Could you check a few things on this model? Use its own coordinates, in mm. A direction names the side the tool comes from. Give positions to 0.01 mm unless a question says otherwise; leave off trailing zeros. Loops run counter-clockwise (first coordinate to the right, second up) from the corner with the lowest first, then second, coordinate; pieces in that order, holes last. Notation, with made-up numbers: M 19,84.5 L 47,84.5 A18 ccw 47,117.5 Z; hole C 24,0 d2. An arc over 180 degrees is marked long. Answer in a Markdown table with one row per item. Add a question column.
Autodesk Inventor part; units mm, degrees
ref_plane "Work Plane1" through (29, 0, 0) normal (0, -1, 0) x (1, 0, 0)
ref_plane "YZ Plane" through (0, 0, 0) normal (1, 0, 0) x (0, 1, 0)
ref_plane "XZ Plane" through (0, 0, 0) normal (0, 1, 0) x (-1, 0, 0)
sketch "Sketch1" plane through (0, 0, 0) normal (0, 0, 1) x (1, 0, 0)
  line L0 (0.2879, 0) -> (6.35, 0)
  line L1 (6.35, 0) -> (6.35, 2.413)
  line L2 (6.35, 2.413) -> (2.1084, 2.413)
  line L3 (2.1084, 2.413) -> (0.0001, 2.413)
  line L4 (0.0001, 2.413) -> (0, 2.413)
  line L5 (0, 2.413) -> (0, 4.5847)
  line L6 (0, 4.5847) -> (-2.5654, 4.5847)
  line L7 (-2.5654, 4.5847) -> (-2.5654, 1.8624)
  line L8 (-2.5654, 1.8624) -> (-0.7874, 1.8624)
  line L9 (-0.7874, 1.8624) -> (0.2879, 0)
  line L10 (-4.3485, 0) -> (8.1331, 0)
  line L11 (0, -0.9169) -> (0, 5.5016)
  line L12 (2.1084, 2.413) -> (0, 2.413) construction
  dimension "d1" = 4.2416
  dimension "d2" = 2.1083
  dimension "d3" = 2.5654
  dimension "d4" = 1.778
  dimension "d5" = 60
  dimension "d6" = 4.826
  dimension "d7" = 4.826
  dimension "d8" = 3.7248
  dimension "d9" = 9.1694
  dimension "d26" = 6.35
revolve "Body" add sketch "Sketch1" angle 360 about axis through (0.2879, 0, 0) along (1, 0, 0) contours L9 L11 L3 L2 L1 L0 | L9 L8 L7 L6 L5 L11
sketch "Sketch2" plane through (-2.5654, 0, 0) normal (-1, 0, 0) x (0, 0, 1)
  circle A0 centre (0, 0) radius 1.8624
  line L0 (0, -6.4186) -> (0, 6.4186)
  line L1 (-6.4186, 0) -> (6.4186, 0)
  line L2 (1.8624, 0) -> (0.9312, -1.6129)
  line L3 (0.9312, -1.6129) -> (-0.9312, -1.6129)
  line L4 (-0.9312, -1.6129) -> (-1.8624, 0)
  line L5 (-1.8624, 0) -> (-0.9312, 1.6129)
  line L6 (-0.9312, 1.6129) -> (0.9312, 1.6129)
  line L7 (0.9312, 1.6129) -> (1.8624, 0)
  point P0 (0, 0)
extrude "Slot" add sketch "Sketch2" against normal up to next contours L7 A0 | A0 L2 | L6 L0 A0 | A0 L0 L3 | L0 L6 A0 | A0 L3 L0 | L4 A0 | A0 L5
fillet "Fillet1" radius 2.0574 1 edges at (-2.5654, -4.5847, 0)
thread "Thread"
chamfer "Chamfer1" distance 0.4724 distance2 0.4724 1 edges at (6.35, -2.413, 0) measured on face at (6.35, -0.2686, 0.7084)
ref_plane "Work Plane1" through (29, 0, 0) normal (0, -1, 0) x (1, 0, 0)
fillet "Fillet2" radius 0.1 1 edges at (0.0001, -2.413, 0)
equation "\"d30\" = R"
equation "\"d17\" = RR"
equation "\"d13\" = GEL"
equation "\"d15\" = -0.5 * SPD + 0.5 * GD"
equation "\"d16\" = GUL"
equation "\"d1\" = GEL"
equation "\"d3\" = KOH"
equation "\"d4\" = INTI"
equation "\"d6\" = GD"
equation "\"d7\" = BDM"
equation "\"d8\" = 1.1547 * SW"
equation "\"d9\" = KOD"
equation "\"d26\" = NLG"
equation "\"GD\" = NND"
equation "\"NLG\" = 6.35"
equation "\"GEL\" = 4.2416"
equation "\"KOD\" = 9.1694"
equation "\"KOH\" = 2.5654"
equation "\"INTI\" = 1.778"
equation "\"GAL\" = 2.1082"
equation "\"GUL\" = 0.47244"
equation "\"BDM\" = NND"
equation "\"SW\" = 3.2258"
equation "\"RR\" = 2.0574"
equation "\"SPD\" = 3.88112"
equation "\"R\" = 0.1"
equation "\"TOA\" = 30deg"
equation "\"GD1\" = SPD"
equation "\"THREADDIA\" = 4.826"
equation "\"KOH1\" = 0.508"
equation "\"NND\" = 4.826"
equation "\"E0\" = 3.72593"
properties part number "ANSI B18.3 - No. 10-32 - 1/4, HSBHCSI" material "Steel, Mild"
Item 1: If we mould it in two halves opening along Y, with no side actions, what happens to faces 1 (the face through (-0.26, -3.64, 2.79)), 2 (the face through (6.35, 0, 0)), 3 (the face through (-2, -1.613, 0))? For each: +Y half, -Y half, draft (parallel to the pull), parting line (faces both ways), or undercut.
Item 2: Suppose I cut it at A-A (x = 4.25). List the corners of the cut face in (y, z) for me, then the cut area to 3 significant figures.
Item 3: For P1, Ø0.9, axis at x = -2, z = 0, coming from the -Y side; P2, Ø1, axis at x = 2, y = -2, coming from the +Z side; P3, Ø1.5, axis at x = -1, y = -2, coming from the +Z side, each with a flat end and sliding along its axis, tell me the tip position at first contact or that it passes through.
Item 4: I need wall thicknesses on L1, parallel to Y at x = -1, z = -0.75; L2, parallel to Z at x = -0.5, y = -0.25; L3, parallel to Y at x = 0.75, z = -0.5. Which ranges of each line are inside material? Lowest first, please.
Item 5: For faces 4 (the face through (-1.6, 0.8, 1.4)), 5 (the face through (0, -1, 3)), 6 (the face through (-2.565, -2, 0)), which set-ups out of +Z, -Z, +X, -X, +Y, -Y let a thin tool reach every point of the face, with its end or its side?
Values found:
| question | item | result |
|---|---|---|
| 1 | face 1 | parting line |
| 1 | face 2 | draft |
| 1 | face 3 | undercut |
| 2 | outline | C 0,0 d4.83 |
| 2 | area | 18.3 mm² |
| 3 | P1 | y = -4.3 |
| 3 | P2 | z = 1.89 |
| 3 | P3 | z = 4.38 |
| 4 | L1 | -4.46 to -1.61, 1.61 to 4.46 |
| 4 | L2 | -4.58 to -1.34, 1.34 to 4.58 |
| 4 | L3 | -2.36 to 2.36 |
| 5 | face 4 | -X |
| 5 | face 5 | +X |
| 5 | face 6 | +Z, -Z, -X, +Y, -Y |
